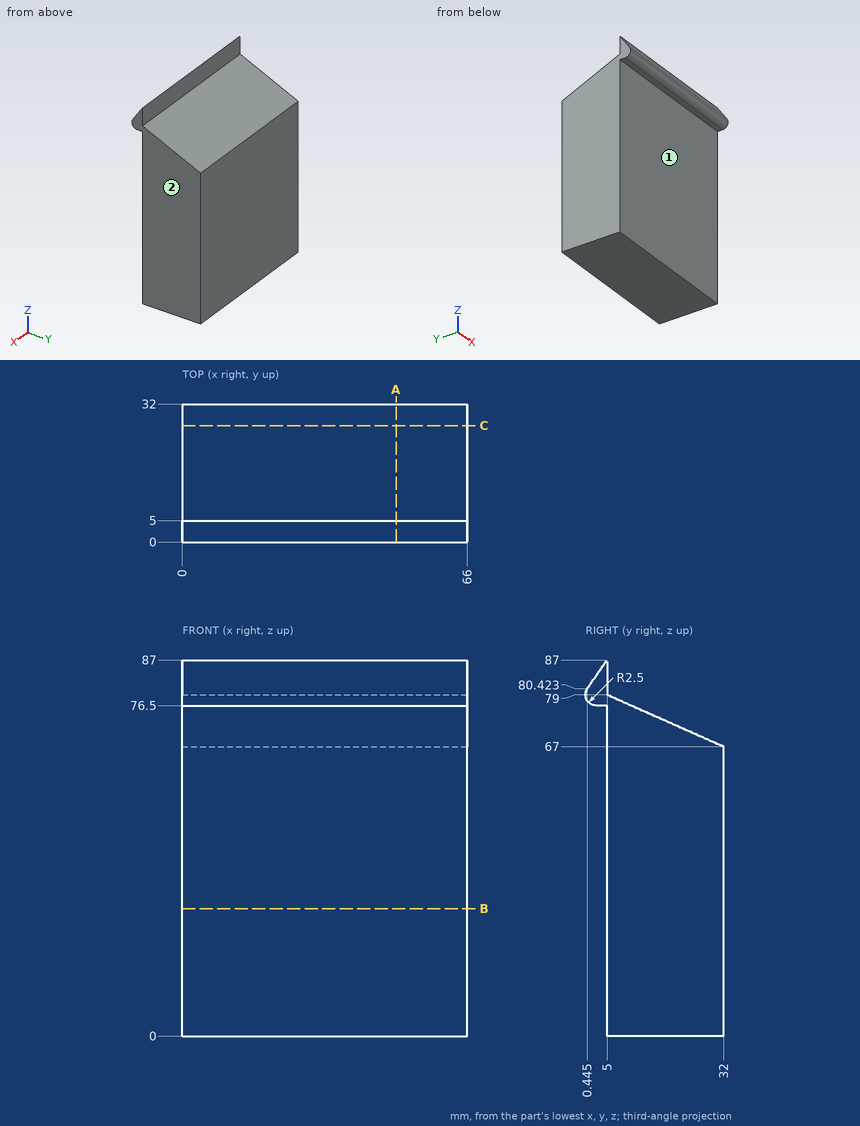
Answer from the drawing. Dimensions are ordinates in mm from the lowest x, y and z of the part. A direction names the side the tool comes from. Give positions to 0.01 mm unless a question says otherwise; leave off trailing zeros. Write each loop counter-clockwise with the first axis right and the second up, starting at its lowest first coordinate (ties: lowest second). Pieces come first, ordered by that corner, then holes. Notation, with made-up numbers: (52.25, 15.5) -> (85.25, 15.5) arc R19 cw to (85.25, 44.5) -> close; hole circle Ø6 at (-30, 65). An arc over 180 degrees is marked (long way). Use a Markdown table: item, result.
(1) Section B-B, the plane z = 29.5 is taken. Determine the outline of the cut face in (x, y).
Return value:
| item | result |
|---|---|
| outline | (0, 5) -> (66, 5) -> (66, 32) -> (0, 32) -> close |
(2) Flat-ended cylindrical pins translate along their axes: P1, Ø0.8, axis at x = 32.5, y = 3.5, coming from the -Z side; P2, Ø8, axis at y = 21, z = 73, coming from the +X side; P3, Ø2, axis at x = 56, z = 52, coming from the -Y side; P4, Ø10, axis at x = 27.5, y = 24, coming from the +Z side. Find the tip coordinate at first contact, or state that the pin passes through.
Return value:
| item | result |
|---|---|
| P1 | z = 76.5 |
| P2 | x = 66 |
| P3 | y = 5 |
| P4 | z = 72.78 |
(3) Section C-C, the plane y = 27 is taken. Determine the outline of the cut face in (x, z).
Return value:
| item | result |
|---|---|
| outline | (0, 0) -> (66, 0) -> (66, 69.22) -> (0, 69.22) -> close |
(4) Find the intervals of material crossed by probe 1 along Y at (x, z) = (28.5, 17); probe 2 along Z at (x, y) = (5.5, 18.5); probe 3 along Z at (x, y) = (49.5, 10), in increasing order. Write a range as from..to.
Return value:
| item | result |
|---|---|
| probe 1 | 5..32 |
| probe 2 | 0..73 |
| probe 3 | 0..76.78 |
(5) Section A-A, the plane x = 49.5 is taken. Determine the outline of the cut face in (y, z) (1 decimal), then the cut area to 3 significant figures.
Return value:
| item | result |
|---|---|
| outline | (0.4, 80.4) arc R2.5 ccw to (2.5, 76.5) -> (5, 76.5) -> (5, 0) -> (32, 0) -> (32, 67) -> (5, 79) -> (5, 87) -> close |
| area | 2,000 mm2 |
(6) For the marked faces 1 and 2, determine the directions among +Z, -Z, +X, -X, +Y, -Y from which every point of the face is accessible in a straight line to the end or side of a thin tool.
Return value:
| item | result |
|---|---|
| face 1 | -Z, +X, -X, -Y |
| face 2 | +Z, -Z, +X, +Y, -Y |
